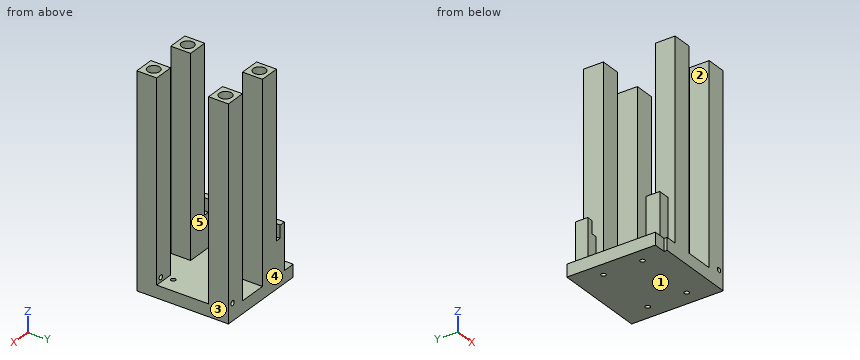
Autodesk Fusion 360 part; units mm, degrees
sketch "Skizze1" plane through (0, 0, 0) normal (0, 0, 1) x (1, 0, 0)
  line L0 (-15.05, 15.05) -> (14.75, 15.05)
  line L1 (14.75, 15.05) -> (14.75, -14.75)
  line L2 (14.75, -14.75) -> (-15.05, -14.75)
  line L3 (-15.05, -14.75) -> (-15.05, 15.05)
  circle A0 centre (-10.41, 6.4) radius 0.75
  circle A1 centre (9.91, 6.4) radius 0.75
  circle A2 centre (-10.41, -6.3) radius 0.75
  circle A3 centre (9.91, -6.3) radius 0.75
  dimension "d1" = 14.75
  dimension "d3" = 14.75
  dimension "d4" = 29.8
  dimension "d5" = 1.5
  dimension "d6" = 1.5
  dimension "d7" = 1.5
  dimension "d8" = 1.5
  dimension "d9" = 20.32
  dimension "d10" = 20.32
  dimension "d11" = 12.7
  dimension "d12" = 12.7
  dimension "d13" = 4.84
  dimension "d14" = 8.65
  dimension "d15" = 4.84
  dimension "d120" = 8.65
extrude "Extrusion1" add sketch "Skizze1" along normal blind 4 contours L0 L1 L2 L3 | A0 | A1 | A2 | A3 makes body 1
sketch "Skizze2" plane through (0, 0, 4) normal (0, 0, 1) x (-1, 0, 0)
  line L0 (15.05, 14.75) -> (-14.75, 14.75)
  line L1 (-14.75, 14.75) -> (-14.75, -15.05)
  line L2 (-14.75, -15.05) -> (15.05, -15.05)
  line L3 (15.05, -15.05) -> (15.05, 14.75)
  circle A0 centre (-3.7, -0.15) radius 9.6
  circle A1 centre (-3.7, -0.15) radius 11.6
  circle A2 centre (-9.91, 6.3) radius 0.75
  line L4 (-14.75, 14.75) -> (15.05, 14.75)
  line L5 (15.05, -15.05) -> (-14.75, -15.05)
  line L6 (15.05, 14.75) -> (11.05, 14.75)
  line L7 (11.05, 14.75) -> (11.05, 13.75)
  line L8 (11.05, 13.75) -> (15.05, 13.75)
  line L9 (15.05, 13.75) -> (15.05, 14.75)
  line L10 (15.05, 14.75) -> (14.05, 14.75)
  line L11 (14.05, 14.75) -> (14.0476, 10.75)
  line L12 (14.0476, 10.75) -> (15.05, 10.75)
  line L13 (15.05, 10.75) -> (15.05, 14.75)
  line L14 (7.35, -15.05) -> (9.05, -15.05)
  line L15 (9.05, -15.05) -> (9.05, 10.35)
  line L16 (9.05, 10.35) -> (7.35, 10.35)
  line L17 (7.35, 10.35) -> (7.35, -15.05)
  line L18 (5.35, -17.05) -> (11.05, -17.05)
  line L19 (11.05, -17.05) -> (11.05, 12.35)
  line L20 (11.05, 12.35) -> (5.35, 12.35)
  line L21 (5.35, 12.35) -> (5.35, -17.05)
  line L22 (5.35, 6.35) -> (11.05, 6.35)
  line L23 (5.35, -11.05) -> (11.05, -11.05)
  line L24 (-14.75, -15.05) -> (-8.2846, -15.05)
  line L25 (-8.2846, -15.05) -> (-8.2846, -8.5846)
  line L26 (-8.2846, -8.5846) -> (-14.75, -8.5846)
  line L27 (-14.75, -8.5846) -> (-14.75, -15.05)
  line L28 (-14.75, 14.75) -> (-8.2846, 14.75)
  line L29 (-8.2846, 14.75) -> (-8.2846, 8.2846)
  line L30 (-8.2846, 8.2846) -> (-14.75, 8.2846)
  line L31 (-14.75, 8.2846) -> (-14.75, 14.75)
  line L32 (7.35, -15.05) -> (0.8846, -15.05)
  line L33 (0.8846, -15.05) -> (0.8846, -8.5846)
  line L34 (0.8846, -8.5846) -> (7.35, -8.5846)
  line L35 (7.35, -8.5846) -> (7.35, -15.05)
  line L36 (0.8846, 14.75) -> (7.35, 14.75)
  line L37 (7.35, 14.75) -> (7.35, 8.2846)
  line L38 (7.35, 8.2846) -> (0.8846, 8.2846)
  line L39 (0.8846, 8.2846) -> (0.8846, 14.75)
  line L40 (9.05, 7.85) -> (11.05, 7.85)
  line L41 (7.35, 8.2846) -> (11.05, 8.2846)
  line L42 (-11.5203, -7.2177) -> (-14.8261, 3.1318)
  line L43 (-11.9705, 6.4686) -> (-11.6289, 6.5777)
  line L44 (-11.6289, 6.5777) -> (-13.2589, 1.4745)
  line L45 (-3.7, -0.15) -> (-14.75, 3.3795)
  line L46 (-3.7, -0.15) -> (-14.75, -3.6795)
  dimension "d18" = 19.2
  dimension "d19" = 2
  dimension "d26" = 14.9
  dimension "d135" = 4
  dimension "d136" = 1
  dimension "d137" = 1
  dimension "d138" = 4
  dimension "d153" = 1.7
  dimension "d154" = 25.4
  dimension "d155" = 2
  dimension "d156" = 4
  dimension "d157" = 4
  dimension "d160" = 6
  dimension "d215" = 11.05
extrude "Extrusion29" cut sketch "Skizze1" along normal blind 4 contours A0 | A1 | A2 | A3 bodies 1
extrude "Extrusion31" add sketch "Skizze2" along normal blind 10.9 separate body contours L15 L16 L17 L37 L41 | L2 L5 L14 L15 L17 L23 L35 makes body 2 at (-7.35, -9.6615, 11.2667) makes body 3 at (-7.35, 12.3833, 7.6333)
extrude "Extrusion32" add sketch "Skizze2" along normal blind 15 contours L15 L16 L19 L20 L37 L41 | L2 L5 L15 L19 L23 | L15 L19 L40 L41 bodies 1 2 3
extrude "Extrusion34" cut sketch "Skizze2" against normal blind 4 contours L0 L3 L4 L6 L8 L9 L10 L11 L13 | L0 L4 L6 L7 L8 L11 bodies 1
extrude "Extrusion35" add sketch "Skizze2" along normal blind 64 contours L0 A1 L4 L20 L21 L36 L37 L38 L39 | L17 L20 L21 L37 L38 | L0 L1 A1 L4 L28 L29 L30 L31 | A1 L38 L39 | A1 L29 L30 | L2 L5 L17 L21 L23 L32 L35 | L2 A1 L5 L21 L32 L33 L34 | L17 L21 L23 L34 L35 | A1 L33 L34 | L1 L2 A1 L5 L24 L25 L26 L27 | A1 L25 L26 bodies 1
sketch "Skizze9" plane through (0, 0, 68) normal (0, 0, 1) x (-1, 0, 0)
  line L0 (-14.75, 8.2846) -> (-8.2846, 8.2846)
  line L1 (-8.2846, 8.2846) -> (-8.2846, 14.75)
  line L2 (-8.2846, 14.75) -> (-14.75, 14.75)
  line L3 (-14.75, 14.75) -> (-14.75, 8.2846)
  line L4 (-14.75, 14.75) -> (-8.2846, 8.2846)
  line L5 (-14.75, 8.2846) -> (-8.2846, 14.75)
  circle A0 centre (-11.5173, 11.5173) radius 2
  dimension "d225" = 4
sketch "Skizze10" plane through (0, 0, 68) normal (0, 0, 1) x (-1, 0, 0)
  line L0 (0.8846, 8.2846) -> (7.35, 8.2846)
  line L1 (7.35, 8.2846) -> (7.35, 14.75)
  line L2 (7.35, 14.75) -> (0.8846, 14.75)
  line L3 (0.8846, 14.75) -> (0.8846, 8.2846)
  line L4 (0.8846, 8.2846) -> (7.35, 14.75)
  line L5 (0.8846, 14.75) -> (7.35, 8.2846)
  circle A0 centre (4.1173, 11.5173) radius 2
  dimension "d226" = 4
sketch "Skizze11" plane through (0, 0, 68) normal (0, 0, 1) x (-1, 0, 0)
  line L0 (7.35, -8.5846) -> (0.8846, -8.5846)
  line L1 (0.8846, -8.5846) -> (0.8846, -15.05)
  line L2 (0.8846, -15.05) -> (7.35, -15.05)
  line L3 (7.35, -15.05) -> (7.35, -8.5846)
  line L4 (0.8846, -8.5846) -> (7.35, -15.05)
  line L5 (0.8846, -15.05) -> (7.35, -8.5846)
  circle A0 centre (4.1173, -11.8173) radius 2
  dimension "d227" = 4
sketch "Skizze12" plane through (0, 0, 68) normal (0, 0, 1) x (-1, 0, 0)
  line L0 (-14.75, -8.5846) -> (-14.75, -15.05)
  line L1 (-14.75, -15.05) -> (-8.2846, -15.05)
  line L2 (-8.2846, -15.05) -> (-8.2846, -8.5846)
  line L3 (-8.2846, -8.5846) -> (-14.75, -8.5846)
  line L4 (-14.75, -8.5846) -> (-8.2846, -15.05)
  line L5 (-14.75, -15.05) -> (-8.2846, -8.5846)
  circle A0 centre (-11.5173, -11.8173) radius 2
  dimension "d228" = 4
extrude "Extrusion36" cut sketch "Skizze10" sketch "Skizze9" sketch "Skizze12" sketch "Skizze11" against normal blind 10 contours L4 L5 A0 | L4 L5 A0 | L4 L5 A0 | L4 L5 A0 of sketch 2 contours L4 L5 A0 | L4 L5 A0 | L4 L5 A0 | L4 L5 A0 of sketch 3 contours L4 L5 A0 | L4 L5 A0 | L4 L5 A0 | L4 L5 A0 of sketch 4 contours L4 L5 A0 | L4 L5 A0 | L4 L5 A0 | L4 L5 A0 bodies 1
sketch "Skizze13" plane through (0, -14.75, 0) normal (0, -1, 0) x (1, 0, 0)
  line L0 (-11.05, 4) -> (-11.05, 0)
  line L1 (-11.05, 0) -> (14.75, 0)
  line L2 (14.75, 0) -> (14.75, 68)
  line L3 (14.75, 68) -> (8.2846, 68)
  line L4 (8.2846, 68) -> (8.2846, 4)
  line L5 (8.2846, 4) -> (-0.8846, 4)
  line L6 (-0.8846, 4) -> (-0.8846, 68)
  line L7 (-0.8846, 68) -> (-7.35, 68)
  line L8 (-7.35, 68) -> (-7.35, 4)
  line L9 (-7.35, 4) -> (-11.05, 4)
  circle A0 centre (12.85, 6) radius 2
  line L10 (14.75, 0) -> (-15.05, 0)
  circle A1 centre (6.35, 6) radius 2
  circle A2 centre (-0.15, 6) radius 2
  circle A3 centre (-6.65, 6) radius 2
  circle A4 centre (-13.15, 6) radius 2
  line L11 (-6.65, 6) -> (-6.65, 5.5)
  circle A5 centre (-6.65, 5.5) radius 1.5
  circle A6 centre (-6.65, 5.5) radius 0.65
  line L12 (12.85, 6) -> (12.85, 5.5)
  circle A7 centre (12.85, 5.5) radius 1.5
  circle A8 centre (12.85, 5.5) radius 0.75
  dimension "d231" = 4
  dimension "d232" = 6
  dimension "d233" = 1.9
  dimension "d236" = -26
  dimension "d237" = 0
  dimension "d240" = 0.5
  dimension "d241" = 3
  dimension "d242" = 1.3
  dimension "d243" = 0.5
  dimension "d244" = 1.5
extrude "Extrusion37" cut sketch "Skizze13" against normal blind 29.8 contours A8 bodies 1
equation "d1 = 29.5 mm / 2"
equation "d3 = 29.5 mm / 2"
equation "d13 = ( 30 mm - 0.8 in ) / 2"
equation "d14 = ( 30 mm - 0.5 in ) / 2"
equation "d15 = ( 30 mm - 0.8 in ) / 2"
equation "d26 = ( 29.8 / 2 ) * 1 mm"
equation "d120 = ( 30 mm - 0.5 in ) / 2"
equation "d215 = ( 22.1 / 2 ) * 1 mm"
Geometry: final body of the model. Coordinates: model frame, mm. Face numbers are marked on the shaded views. A direction names the side the tool comes from. Coordinates: 2 decimals unless noted, no trailing zeros. Order: outer loops, then holes, each group sorted by start corner. A loop starts at its lowest first (then second) coordinate and runs counter-clockwise, first axis right, second up. Notation, with made-up numbers: M -34,-39 L 1,-39 A26 ccw 1,-10 Z; hole C -12,49.25 d10. An arc over 180 degrees is marked long. One line per question, with ' | ' between items. Start each with the question number.
Item 1: Ray query, probe 1 along Y at (x, z) = (-10.41, 3.2); probe 2 along Y at (x, z) = (13.75, 53); probe 3 along Y at (x, z) = (12, 64.5). Return the intervals inside material, ascending. Write a range as [from, to].
Item 2: Cut plane A-A, the plane z = 5.5. Count the separate pieces of the cut face and the enclosed holes in it, then the cut area to 3 significant figures.
Item 3: Pin query (flat end, axial travel): pin 1 Ø5 at (y, z) = (-8, 12.5) entering from +X; pin 2 Ø2 at (y, z) = (14, 14.5) entering from -X; pin 3 Ø3 at (x, y) = (-9.5, -10.5) entering from +Z; pin 4 Ø0.9 at (x, y) = (-8.5, 12.5) entering from +Z. Return the tip coordinate at first contact, or that it passes through.
Item 4: Draft query along Y for the marked faces 3, 4 and 5. Return one class per face: released by +Y, released by -Y, zero draft, split by the parting line, or undercut.
Item 5: Cut plane D-D, the plane x = -5. Return the cut outline in (y, z).
Item 6: Cut plane C-C, the plane z = 60. Return the cut outline in (x, y), then the cut area to 3 significant figures.
Item 7: Set-up query: the marked faces 1 and 2. Return all of +Z, -Z, +X, -X, +Y, -Y with unobstructed straight access to the full face (end or side cutting, diameter ignored); none if empty.
Item 8: Cut plane B-B, the plane y = 6.4. Return the cut outline in (x, z).
A:
1) probe 1: y = [-14.75, -7.05], [-5.55, 5.65], [7.15, 15.05] | probe 2: y = [-14.75, -8.28], [8.58, 15.05] | probe 3: y = [-14.75, -13.46], [-9.58, -8.28], [8.58, 9.88], [13.76, 15.05]
2) separate pieces: 6 | enclosed holes: 0 | area: 179 mm2
3) pin 1: stops at x = 14.75 | pin 2: stops at x = -11.05 | pin 3: stops at z = 19 | pin 4: stops at z = 14.9
4) face 3: zero draft | face 4: released by +Y | face 5: undercut
5) outline: M -14.75,0 L 15.05,0 L 15.05,68 L 13.61,68 L 13.61,58 L 10.02,58 L 10.02,68 L 8.58,68 L 8.58,4 L -8.28,4 L -8.28,68 L -9.72,68 L -9.72,58 L -13.31,58 L -13.31,68 L -14.75,68 Z
6) outline: M -7.35,-14.75 L -0.88,-14.75 L -0.88,-8.28 L -7.35,-8.28 Z; M -7.35,8.58 L -0.88,8.58 L -0.88,15.05 L -7.35,15.05 Z; M 8.28,-14.75 L 14.75,-14.75 L 14.75,-8.28 L 8.28,-8.28 Z; M 8.28,8.58 L 14.75,8.58 L 14.75,15.05 L 8.28,15.05 Z; hole C -4.12,-11.52 d4; hole C -4.12,11.82 d4; hole C 11.52,-11.52 d4; hole C 11.52,11.82 d4 | area: 117 mm2
7) face 1: -Z, +X, -X, +Y, -Y | face 2: +Z, +Y, -Y
8) outline: M -15.05,0 L -11.16,0 L -11.16,4 L -15.05,4 Z; M -9.66,0 L 9.16,0 L 9.16,4 L -9.66,4 Z; M 10.66,0 L 14.75,0 L 14.75,4 L 10.66,4 Z
